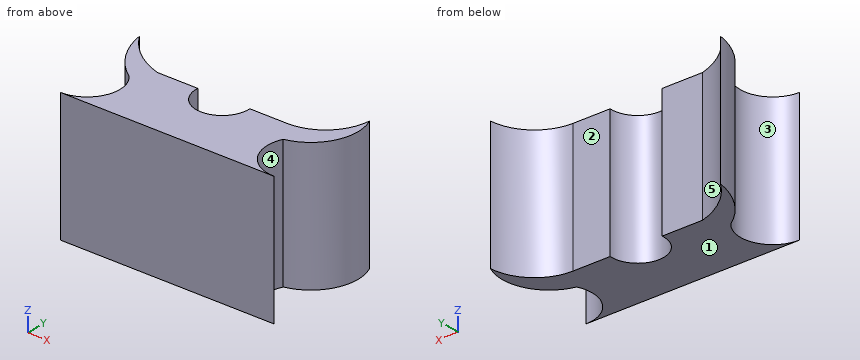
```python
from build123d import *

# Parameters (mm, degrees)
F1_DEPTH = 49.9999


with BuildPart() as f1:
    # F0 (on Top) → F1 (new body)
    with BuildSketch(Plane.XY):
        with BuildLine():
            ThreePointArc((-33.665815, 20.741972), (-31.690377, 7.338264), (-43.079478, 0))
            Line((-43.079478, 0), (-24.252152, 0))
            Line((-24.252152, 0), (39.250193, 0))
            ThreePointArc((39.250193, 0), (27.63624, 6.333119), (26.670001, 19.526249))
            ThreePointArc((26.670001, 19.526249), (38.969207, 29.094689), (39.250193, 44.675015))
            ThreePointArc((39.250193, 44.675015), (33.582753, 32.751227), (21.301444, 27.90705))
            Line((21.301444, 27.90705), (6.903135, 27.90705))
            ThreePointArc((6.903135, 27.90705), (-3.09687, 17.145785), (-13.096876, 27.90705))
            Line((-13.096876, 27.90705), (-28.698456, 27.90705))
            ThreePointArc((-28.698456, 27.90705), (-39.287504, 33.288324), (-47.227875, 42.122154))
            ThreePointArc((-47.227875, 42.122154), (-42.649199, 30.035047), (-33.665815, 20.741972))
        make_face()
    extrude(amount=F1_DEPTH)


solid = f1.part
```
Could you check a few things on this model? Use its own coordinates, in mm. Face numbers are marked on the shaded views. A direction names the side the tool comes from. Round coordinates to 2 decimals unless told otherwise and drop trailing zeros. Write each loop counter-clockwise with the first axis right and the second up, starting at its lowest first coordinate (ties: lowest second). Pieces come first, ordered by that corner, then holes. Notation, with made-up numbers: M 24.25,-5 L 29.25,-5 A20 cw 29.25,0 Z; hole C -32.5,66 d6. An arc over 180 degrees is marked long. Answer in a Markdown table with one row per item. Add a question column.
Q1. On a 3-axis mill with a long thin cutter (end or side, diameter ignored), from which of +Z, -Z, +X, -X, +Y, -Y can I reach the whole of each face in a straight line? I mean the marked faces 4 and 5. Say none if no direction works.
Q2. Imagine slicing it at B-B (y = 39). Please give me the cut outline in (x, z).
Q3. If we mould it in two halves opening along X, with no side actions, what happens to the marked faces 1, 2 and 3? For each: +X half, -X half, draft (parallel to the pull), parting line (faces both ways), or undercut.
Q4. Will these pins go through, and if not, where does the flat tip stop? pin 1 Ø6 at (y, z) = (17.5, 45) entering from -X; pin 2 Ø4.5 at (x, z) = (-21.5, 29.5) entering from +Y; pin 3 Ø5 at (y, z) = (36.5, 16.5) entering from -X.
Q5. Imagine slicing it at A-A (z = 19). Please give me the cut outline in (x, y).
Q6. If I drill on line 1 (Y direction, x = 21, z = 30); line 2 (Y direction, x = 28.5, z = 16); line 3 (X direction, y = 19, z = 4), over which ranges is the centre line in solid material (lowest first)? Write a range as from..to.
Q7. Imagine slicing it at C-C (x = -36). Please give me the cut outline in (y, z), then the cut area to 3 significant figures.
Q8. Imagine slicing it at D-D (x = 11). Please give me the cut outline in (y, z).
Values:
| question | item | result |
|---|---|---|
| 1 | face 4 | +Z, -Z, +X |
| 1 | face 5 | +Z, -Z, +Y |
| 2 | outline | M -46.57,0 L -45.06,0 L -45.06,50 L -46.57,50 Z; M 37.92,0 L 40.79,0 L 40.79,50 L 37.92,50 Z |
| 3 | face 1 | draft |
| 3 | face 2 | undercut |
| 3 | face 3 | -X half |
| 4 | pin 1 | x = -33.46 |
| 4 | pin 2 | y = 27.91 |
| 4 | pin 3 | x = -46.57 |
| 5 | outline | M -47.23,42.12 A32.03 ccw -33.67,20.74 A12.51 cw -43.08,0 L 39.25,0 A13.82 cw 26.67,19.53 A18.07 ccw 39.25,44.68 A17.99 cw 21.3,27.91 L 6.9,27.91 A10.03 cw long -13.1,27.91 L -28.7,27.91 A32.42 cw Z |
| 6 | line 1 | 0..27.91 |
| 6 | line 2 | 0..5.14, 20.03..29.41 |
| 6 | line 3 | -32.39..-8.91, 2.71..26.44 |
| 7 | outline | M 0,0 L 2.2,0 L 2.2,50 L 0,50 Z; M 22.5,0 L 31.07,0 L 31.07,50 L 22.5,50 Z |
| 7 | area | 539 mm^2 |
| 8 | outline | M 0,0 L 27.91,0 L 27.91,50 L 0,50 Z |
